Can you work these out from the model? Positions are in its coordinate system, mm. Coordinates: 2 decimals unless noted, no trailing zeros. Order: outer loops, then holes, each group sorted by start corner. A loop starts at its lowest first (then second) coordinate and runs counter-clockwise, first axis right, second up. Notation, with made-up numbers: (44.5, -37.5) -> (61.5, -37.5) arc R32 cw to (61.5, -10.5) -> close; hole circle Ø7 at (57.5, -0.75). An arc over 180 degrees is marked (long way). Write item = value, one per line. Start each with the question number.
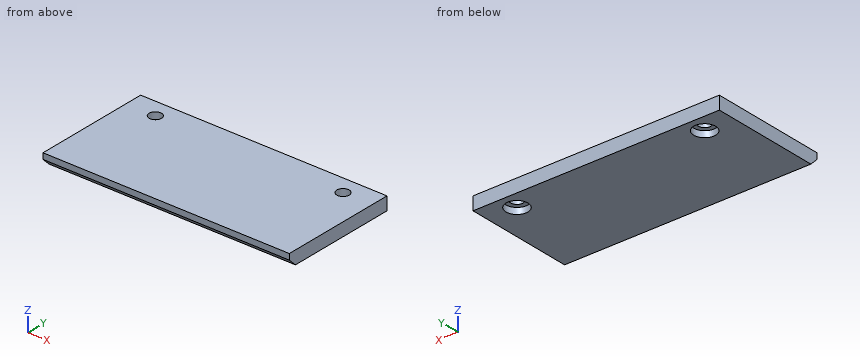
from build123d import *

# Parameters (mm, degrees)
SKETCH1_W                                        = 133.35
SKETCH1_H                                        = 63.5
BOSS_EXTRUDE1_DEPTH                              = 3.5687
CUT_EXTRUDE1_DEPTH                               = 134.35
CBORE_FOR_1_4_BUTTON_HEAD_CAP_SCREW1_D           = 6.7564
CBORE_FOR_1_4_BUTTON_HEAD_CAP_SCREW1_CBORE_D     = 11.90752
CBORE_FOR_1_4_BUTTON_HEAD_CAP_SCREW1_CBORE_DEPTH = 3.3528


with BuildPart() as part:
    # Sketch1 → Boss-Extrude1 (new body, symmetric)
    with BuildSketch(Plane.XY):
        Rectangle(SKETCH1_W, SKETCH1_H)
    extrude(amount=BOSS_EXTRUDE1_DEPTH, both=True)

    # Sketch2 → Cut-Extrude1 (cut, through all)
    with BuildSketch(Plane.ZY.offset(66.675)):
        Polygon((0.3937, -31.75), (-3.5687, -27.7876), (-3.5687, -31.75), align=None)
    extrude(amount=-CUT_EXTRUDE1_DEPTH, mode=Mode.SUBTRACT)

    # CBORE for 1/4 Button Head Cap Screw1 (through all)
    with Locations(Plane(origin=(0, 0, -3.5687), x_dir=(-1, 0, 0), z_dir=(0, 0, -1))):
        with Locations((-50.8, 22.225), (50.8, 22.225)):
            CounterBoreHole(CBORE_FOR_1_4_BUTTON_HEAD_CAP_SCREW1_D / 2, CBORE_FOR_1_4_BUTTON_HEAD_CAP_SCREW1_CBORE_D / 2, CBORE_FOR_1_4_BUTTON_HEAD_CAP_SCREW1_CBORE_DEPTH)


solid = part.part
(1) If I drill on L1, parallel to Y at x = -50.8, z = 2.05; L2, parallel to X at y = 25, z = -1 (1 decimal); L3, parallel to X at y = 21, z = -3 (3 decimals), over which ranges is the centre line in solid material (lowest first)? Write a range as from..to.
(2) For P1, Ø3.5, axis at x = -53, y = 23.5, coming from the -Z side; P2, Ø19, axis at x = 50.8, y = 22.225, coming from the -Z side; P3, Ø4, axis at x = 50.8, y = 22.225, coming from the -Z side, each with a flat end and sliding along its axis, tell me the tip position at first contact or that it passes through.
(3) Imagine slicing it at B-B (x = 5.5). Write out the boundary of the cut face in (y, z).
(4) Imagine slicing it at A-A (x = 50.8). Write out the boundary of the cut face in (y, z), plus the area to 3 significant figures.
Result set:
q1.L1 = -31.75..18.85, 25.6..31.75
q1.L2 = -66.7..-56.1, -45.5..45.5, 56.1..66.7
q1.L3 = -66.675..-56.626, -44.974..44.974, 56.626..66.675
q2.P1 = -0.22
q2.P2 = -3.57
q2.P3 = through
q3.outline = (-31.75, 0.39) -> (-27.79, -3.57) -> (31.75, -3.57) -> (31.75, 3.57) -> (-31.75, 3.57) -> close
q4.outline = (-31.75, 0.39) -> (-27.79, -3.57) -> (16.27, -3.57) -> (16.27, -0.22) -> (18.85, -0.22) -> (18.85, 3.57) -> (-31.75, 3.57) -> close; (25.6, -0.22) -> (28.18, -0.22) -> (28.18, -3.57) -> (31.75, -3.57) -> (31.75, 3.57) -> (25.6, 3.57) -> close
q4.area = 380 mm2
